For this review, take the finished solid that the model builds, in its own axes (mm). Face numbers are marked on the shaded views. Round coordinates to 2 decimals unless told otherwise and drop trailing zeros. Order: outer loops, then holes, each group sorted by start corner. A loop starts at its lowest first (then second) coordinate and runs counter-clockwise, first axis right, second up.
```python
from build123d import *

# Parameters (mm, degrees)
SKETCH1_W           = 42
SKETCH1_H           = 88
BOSS_EXTRUDE1_DEPTH = 2
BOSS_EXTRUDE2_DEPTH = 77
SKETCH3_R           = 2.75
BOSS_EXTRUDE3_DEPTH = 4
FILLET1_R           = 0.5
CHAMFER3_SIZE       = 0.25


with BuildPart() as part:
    # Sketch1 → Boss-Extrude1 (new body)
    with BuildSketch(Plane(origin=(0, 0, 0), x_dir=(1, 0, 0), z_dir=(0, 1, 0))):
        Rectangle(SKETCH1_W, SKETCH1_H)
    extrude(amount=BOSS_EXTRUDE1_DEPTH)

    # Sketch2 → Boss-Extrude2 (add)
    with BuildSketch(Plane.XY.offset(44)):
        Polygon((14.5, 2), (16, 5.535533906), (19, 5.535533906), (17.232233047, 3.767766953), (19, 2), align=None)
    boss_extrude2 = extrude(amount=-BOSS_EXTRUDE2_DEPTH)

    # Mirror1: Boss-Extrude2 across plane
    add(boss_extrude2.mirror(Plane(origin=(0, 0, 0), x_dir=(0, 0, 1), z_dir=(1, 0, 0))))

    # Sketch3 → Boss-Extrude3 (add)
    with BuildSketch(Plane(origin=(0, 2, 0), x_dir=(1, 0, 0), z_dir=(0, 1, 0))):
        with Locations(Location((-9, -41.25, 0), (0, 0, 270))):
            Circle(SKETCH3_R)
        with Locations(Location((8, -41.25, 0), (0, 0, 270))):
            Circle(SKETCH3_R)
        with Locations(Location((8, 3.75, 0), (0, 0, 270))):
            Circle(SKETCH3_R)
        with Locations(Location((-9, 3.75, 0), (0, 0, 270))):
            Circle(SKETCH3_R)
    extrude(amount=BOSS_EXTRUDE3_DEPTH)

    # Fillet1
    fillet1_edges = [part.edges().sort_by_distance(p)[0] for p in [
        (0, 0, -44),
    ]]
    fillet(fillet1_edges, radius=FILLET1_R)

    # Chamfer3
    chamfer3_edges = [part.edges().sort_by_distance(p)[0] for p in [
        (18.116116524, 4.651650429, -33),
        (18.116116524, 2.883883476, -33),
        (18.116116524, 2.883883476, 44),
        (18.116116524, 4.651650429, 44),
        (-18.116116524, 2.883883476, 44),
        (-18.116116524, 4.651650429, 44),
        (-18.116116524, 2.883883476, -33),
        (-18.116116524, 4.651650429, -33),
    ]]
    chamfer(chamfer3_edges, length=CHAMFER3_SIZE)


solid = part.part
```
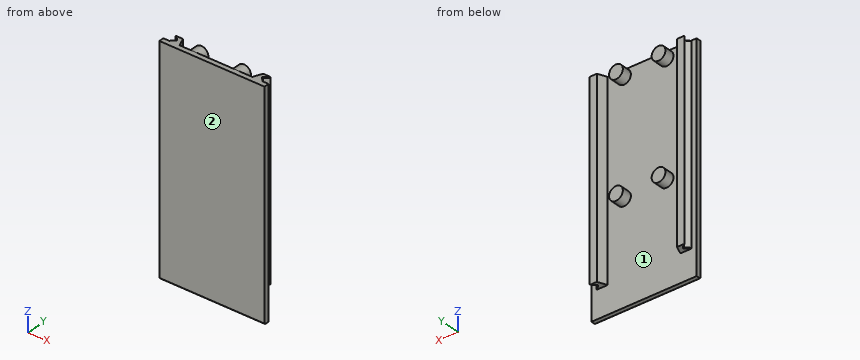
Q1. Take a section at C-C, the plane z = 28.5. State the section outline as (x, y) points.
Q2. Mouldability with a two-part tool opening along Z and no side actions: class the marked faces 1 and 2 as +Z half, -Z half, draft (parallel to the pull), parting line (faces both ways), or undercut.
Q3. Clearance check with flat-ended pins moving along their axes: pin 1 (5 mm diameter, centred on x = 4.5, z = 12, fed in from +Y); pin 2 (2.5 mm diameter, centred on x = 18, z = 22, fed in from +Y); pin 3 (1.8 mm diameter, centred on x = 16, y = 4, fed in from -Z). State where each tip first meets the part, or that it passes through.
Q4. Take a section at A-A, the plane z = 41.25. State the section outline as (x, y) points.
Q5. Take a section at B-B, the plane x = 0. State the section outline as (y, z) points, plus the area to 3 significant figures.
Q6. Wall thickness on line 1 (Y direction, x = -7, z = -19.5); line 2 (Z direction, x = 7, y = 3.4); line 3 (X direction, y = 5.4, z = -9): over which ranges is each line inside the solid? List them lowest first.
Working result:
1. outline: (-21, 0) - (21, 0) - (21, 2) - (19, 2) - (17.23, 3.77) - (19, 5.54) - (16, 5.54) - (14.5, 2) - (-14.5, 2) - (-16, 5.54) - (-19, 5.54) - (-17.23, 3.77) - (-19, 2) - (-21, 2) - close
2. face 1: undercut
2. face 2: draft
3. pin 1: stops at y = 2
3. pin 2: stops at y = 5.54
3. pin 3: stops at z = -33
4. outline: (-21, 0) - (21, 0) - (21, 2) - (19, 2) - (17.23, 3.77) - (19, 5.54) - (16, 5.54) - (14.5, 2) - (10.75, 2) - (10.75, 6) - (5.25, 6) - (5.25, 2) - (-6.25, 2) - (-6.25, 6) - (-11.75, 6) - (-11.75, 2) - (-14.5, 2) - (-16, 5.54) - (-19, 5.54) - (-17.23, 3.77) - (-19, 2) - (-21, 2) - close
5. outline: (0, -43.5) arc R0.5 ccw to (0.5, -44) - (2, -44) - (2, 44) - (0, 44) - close
5. area: 176 mm2
6. line 1: y = 0 to 2
6. line 2: z = -6.31 to -1.19, 38.69 to 43.81
6. line 3: x = -18.86 to -15.94, 15.94 to 18.86
